```python
from build123d import *

# Parameters (mm, degrees)
SKETCH_1_R          = 1.6
EXTRUDE_1_DEPTH     = 3
SKETCH_5_W          = 8.427610272
SKETCH_5_H          = 29.562823711
CUT_EXTRUDE_4_DEPTH = 10
SKETCH_7_W          = 55.144779456
SKETCH_7_H          = 10
CUT_EXTRUDE_1_DEPTH = 100
CUT_EXTRUDE_5_DEPTH = 100
CUT_EXTRUDE_6_DEPTH = 100
FILLET_3_R          = 3
SKETCH_10_W         = 2
SKETCH_10_H         = 2
SKETCH_10_H_2       = 11
SKETCH_10_R         = 1.5
CUT_EXTRUDE_7_DEPTH = 10
SKETCH_11_R         = 11
CUT_EXTRUDE_8_DEPTH = 10


with BuildPart() as part:
    # 草图1 → 凸台-拉伸1 (new body)
    with BuildSketch(Plane(origin=(0, 0, 0), x_dir=(1, 0, 0), z_dir=(0, 1, 0))):
        Polygon((-1, -77.5), (-40, -77.5), (-40, -235.15), (110, -235.15), (110, -77.5), (71, -77.5), (71, -47.937176289), (113.89906921, -47.937176289), (113.89906921, 47.937176289), (71, 47.937176289), (71, 77.5), (110, 77.5), (110, 235.15), (-40, 235.15), (-40, 77.5), (-1, 77.5), (-1, 47.937176289), (-43.89906921, 47.937176289), (-43.89906921, -47.937176289), (-1, -47.937176289), align=None)
        with Locations(Location((48.025, -63.59, 0), (0, 0, 90))):
            Circle(SKETCH_1_R, mode=Mode.SUBTRACT)
        with Locations(Location((58.025, -63.59, 0), (0, 0, 90))):
            Circle(SKETCH_1_R, mode=Mode.SUBTRACT)
        with Locations(Location((58.025, 63.41, 0), (0, 0, 90))):
            Circle(SKETCH_1_R, mode=Mode.SUBTRACT)
        with Locations(Location((48.025, 63.41, 0), (0, 0, 90))):
            Circle(SKETCH_1_R, mode=Mode.SUBTRACT)
        with Locations(Location((11.975, -63.59, 0), (0, 0, 270))):
            Circle(SKETCH_1_R, mode=Mode.SUBTRACT)
        with Locations(Location((21.975, -63.59, 0), (0, 0, 270))):
            Circle(SKETCH_1_R, mode=Mode.SUBTRACT)
        with Locations(Location((21.975, 63.41, 0), (0, 0, 270))):
            Circle(SKETCH_1_R, mode=Mode.SUBTRACT)
        with Locations(Location((11.975, 63.41, 0), (0, 0, 270))):
            Circle(SKETCH_1_R, mode=Mode.SUBTRACT)
        with BuildLine():
            Line((30.075, -69.59), (30.075, -66.41))
            ThreePointArc((30.075, -66.41), (28.475, -64.81), (26.875, -66.41))
            Line((26.875, -66.41), (18.125, -66.41))
            ThreePointArc((18.125, -66.41), (16.525, -64.81), (14.925, -66.41))
            Line((14.925, -66.41), (14.925, -69.59))
            ThreePointArc((14.925, -69.59), (16.525, -71.19), (18.125, -69.59))
            Line((18.125, -69.59), (26.875, -69.59))
            ThreePointArc((26.875, -69.59), (28.475, -71.19), (30.075, -69.59))
        make_face(mode=Mode.SUBTRACT)
        with BuildLine():
            Line((43.125, 69.59), (51.875, 69.59))
            ThreePointArc((51.875, 69.59), (53.475, 71.19), (55.075, 69.59))
            Line((55.075, 69.59), (55.075, 66.41))
            ThreePointArc((55.075, 66.41), (53.475, 64.81), (51.875, 66.41))
            Line((51.875, 66.41), (43.125, 66.41))
            ThreePointArc((43.125, 66.41), (41.525, 64.81), (39.925, 66.41))
            Line((39.925, 66.41), (39.925, 69.59))
            ThreePointArc((39.925, 69.59), (41.525, 71.19), (43.125, 69.59))
        make_face(mode=Mode.SUBTRACT)
        with BuildLine():
            Line((55.075, -69.59), (55.075, -66.41))
            ThreePointArc((55.075, -66.41), (53.475, -64.81), (51.875, -66.41))
            Line((51.875, -66.41), (43.125, -66.41))
            ThreePointArc((43.125, -66.41), (41.525, -64.81), (39.925, -66.41))
            Line((39.925, -66.41), (39.925, -69.59))
            ThreePointArc((39.925, -69.59), (41.525, -71.19), (43.125, -69.59))
            Line((43.125, -69.59), (51.875, -69.59))
            ThreePointArc((51.875, -69.59), (53.475, -71.19), (55.075, -69.59))
        make_face(mode=Mode.SUBTRACT)
        with BuildLine():
            Line((14.925, 69.59), (14.925, 66.41))
            ThreePointArc((14.925, 66.41), (16.525, 64.81), (18.125, 66.41))
            Line((18.125, 66.41), (26.875, 66.41))
            ThreePointArc((26.875, 66.41), (28.475, 64.81), (30.075, 66.41))
            Line((30.075, 66.41), (30.075, 69.59))
            ThreePointArc((30.075, 69.59), (28.475, 71.19), (26.875, 69.59))
            Line((26.875, 69.59), (18.125, 69.59))
            ThreePointArc((18.125, 69.59), (16.525, 71.19), (14.925, 69.59))
        make_face(mode=Mode.SUBTRACT)
    extrude(amount=EXTRUDE_1_DEPTH)

    # 草图5 → 切除-拉伸4 (cut)
    with BuildSketch(Plane.XZ):
        with Locations((66.786194864, 62.718588145)):
            Rectangle(SKETCH_5_W, SKETCH_5_H)
        with Locations((3.213805136, 62.718588145)):
            Rectangle(SKETCH_5_W, SKETCH_5_H)
        with Locations((3.213805136, -62.718588145)):
            Rectangle(SKETCH_5_W, SKETCH_5_H)
        with Locations((66.786194864, -62.718588145)):
            Rectangle(SKETCH_5_W, SKETCH_5_H)
    extrude(amount=-CUT_EXTRUDE_4_DEPTH, mode=Mode.SUBTRACT)

    # 草图7 → 切除-拉伸-薄壁1 (cut)
    with BuildSketch(Plane(origin=(0, 0, 0), x_dir=(-1, 0, 0), z_dir=(0, -1, 0))):
        with Locations((-35, -55.277176289)):
            Rectangle(SKETCH_7_W, SKETCH_7_H)
        Polygon((-113.89906921, -0.33), (-113.89906921, 47.607176289), (-62.572389728, 47.607176289), (-62.572389728, 49.947176289), (-7.427610272, 49.947176289), (-7.427610272, 47.607176289), (43.89906921, 47.607176289), (43.89906921, -0.33), (33.89906921, -0.33), (33.89906921, 37.607176289), (-17.427610272, 37.607176289), (-17.427610272, 39.947176289), (-52.572389728, 39.947176289), (-52.572389728, 37.607176289), (-103.89906921, 37.607176289), (-103.89906921, -0.33), align=None)
    extrude(amount=-CUT_EXTRUDE_1_DEPTH, mode=Mode.SUBTRACT)


with BuildPart() as cut_extrude_1_piece_1:
    # of the separate pieces the step leaves, piece 1, a body of its own (cut_extrude_1_pieces)
    add(part.part.solids().sort_by_distance((7.427610272, 0, -77.5))[0])

    # 草图9 → 切除-拉伸6 (cut)
    with BuildSketch(Plane.XZ):
        Polygon((-40, -102.5), (110, -102.5), (124.211694431, -119.691261336), (154.987235789, -211.57345947), (124.211694431, -286.861832075), (-63.673505757, -270.701496299), (-75.556105593, -182.770257517), (-74.082044988, -165.632360403), align=None)
    extrude(amount=-CUT_EXTRUDE_6_DEPTH, mode=Mode.SUBTRACT)

    # 圆角3
    fillet_3_edges = [cut_extrude_1_piece_1.edges().sort_by_distance(p)[0] for p in [
        (110, 1.5, -77.5),
        (-40, 1.5, -77.5),
        (62.572389728, 1.5, -77.5),
        (7.427610272, 1.5, -77.5),
        (-40, 1.5, -102.5),
        (110, 1.5, -102.5),
        (7.427610272, 1.5, -49.947176289),
        (62.572389728, 1.5, -49.947176289),
    ]]
    fillet(fillet_3_edges, radius=FILLET_3_R)

    # 草图10 → 切除-拉伸7 (cut)
    with BuildSketch(Plane.XZ):
        with BuildLine():
            ThreePointArc((-35, -84.5), (-34, -83.5), (-35, -82.5))
            Line((-35, -82.5), (-35, -84.5))
        make_face()
        with BuildLine():
            Line((-37, -84.5), (-37, -82.5))
            ThreePointArc((-37, -82.5), (-38, -83.5), (-37, -84.5))
        make_face()
        with Locations((-36, -83.5)):
            Rectangle(SKETCH_10_W, SKETCH_10_H)
        with Locations((-36, -90)):
            Rectangle(SKETCH_10_W, SKETCH_10_H_2)
        with Locations((-36, -96.5)):
            Rectangle(SKETCH_10_W, SKETCH_10_H)
        with BuildLine():
            Line((-37, -97.5), (-37, -95.5))
            ThreePointArc((-37, -95.5), (-38, -96.5), (-37, -97.5))
        make_face()
        with BuildLine():
            ThreePointArc((-35, -97.5), (-34, -96.5), (-35, -95.5))
            Line((-35, -95.5), (-35, -97.5))
        make_face()
        with Locations(Location((-31.5, -95, 0), (0, 0, 270))):
            Circle(SKETCH_10_R)
        with Locations(Location((-31.5, -85, 0), (0, 0, 270))):
            Circle(SKETCH_10_R)
        with BuildLine():
            ThreePointArc((107, -97.5), (108, -96.5), (107, -95.5))
            Line((107, -95.5), (107, -97.5))
        make_face()
        with Locations((106, -96.5)):
            Rectangle(SKETCH_10_W, SKETCH_10_H)
        with BuildLine():
            Line((105, -97.5), (105, -95.5))
            ThreePointArc((105, -95.5), (104, -96.5), (105, -97.5))
        make_face()
        with Locations((106, -90)):
            Rectangle(SKETCH_10_W, SKETCH_10_H_2)
        with BuildLine():
            ThreePointArc((107, -84.5), (108, -83.5), (107, -82.5))
            Line((107, -82.5), (107, -84.5))
        make_face()
        with Locations((106, -83.5)):
            Rectangle(SKETCH_10_W, SKETCH_10_H)
        with BuildLine():
            Line((105, -84.5), (105, -82.5))
            ThreePointArc((105, -82.5), (104, -83.5), (105, -84.5))
        make_face()
        with Locations(Location((101.5, -85, 0), (0, 0, 270))):
            Circle(SKETCH_10_R)
        with Locations(Location((101.5, -95, 0), (0, 0, 270))):
            Circle(SKETCH_10_R)
    extrude(amount=-CUT_EXTRUDE_7_DEPTH, mode=Mode.SUBTRACT)

    # 草图11 → 切除-拉伸8 (cut)
    with BuildSketch(Plane.XZ):
        with Locations(Location((35, -86.015496457, 0), (0, 0, 270))):
            Circle(SKETCH_11_R)
    extrude(amount=-CUT_EXTRUDE_8_DEPTH, mode=Mode.SUBTRACT)


with BuildPart() as cut_extrude_1_piece_2:
    # of the separate pieces the step leaves, piece 2, a body of its own (cut_extrude_1_pieces)
    add(part.part.solids().sort_by_distance((-40, 0, 77.5))[0])


with BuildPart() as cut_extrude_1_piece_3:
    # of the separate pieces the step leaves, piece 3, a body of its own (cut_extrude_1_pieces)
    add(part.part.solids().sort_by_distance((7.427610272, 0, 50.277176289))[0])


with BuildPart() as cut_extrude_1_piece_4:
    # of the separate pieces the step leaves, piece 4, a body of its own (cut_extrude_1_pieces)
    add(part.part.solids().sort_by_distance((113.89906921, 0, -47.607176289))[0])


with BuildPart() as cut_extrude_1_piece_5:
    # of the separate pieces the step leaves, piece 5, a body of its own (cut_extrude_1_pieces)
    add(part.part.solids().sort_by_distance((-43.89906921, 0, -47.937176289))[0])


with BuildPart() as cut_extrude_5_tool:
    # 草图8 → 切除-拉伸5 (new body)
    with BuildSketch(Plane(origin=(0, 0, 0), x_dir=(-1, 0, 0), z_dir=(0, -1, 0))):
        Polygon((78.212914253, 60.385355647), (0, 54.326624312), (-4.481912928, 51.672567956), (-7.938908088, 48.761414138), (-49.331876445, 46.578048774), (-63.52375131, 48.761414138), (-79.080229528, 55.85735157), (-126.563695568, 60.385355647), (-136.561762242, 25.020008622), (-185.509289936, -177.467896247), (-114.798778659, -331.741539621), (230.896230576, -266.427705394), (230.896230576, -108.933419225), (223.681342993, -70.746247105), align=None)
    extrude(amount=-CUT_EXTRUDE_5_DEPTH)


with BuildPart() as cut_extrude_1_piece_2_1:
    add(cut_extrude_1_piece_2.part)

    # 切除-拉伸5: cut by cut_extrude_5_tool
    add(cut_extrude_5_tool.part, mode=Mode.SUBTRACT)


with BuildPart() as cut_extrude_1_piece_3_1:
    add(cut_extrude_1_piece_3.part)

    # 切除-拉伸5: cut by cut_extrude_5_tool
    add(cut_extrude_5_tool.part, mode=Mode.SUBTRACT)


with BuildPart() as cut_extrude_1_piece_4_1:
    add(cut_extrude_1_piece_4.part)

    # 切除-拉伸5: cut by cut_extrude_5_tool
    add(cut_extrude_5_tool.part, mode=Mode.SUBTRACT)


with BuildPart() as cut_extrude_1_piece_5_1:
    add(cut_extrude_1_piece_5.part)

    # 切除-拉伸5: cut by cut_extrude_5_tool
    add(cut_extrude_5_tool.part, mode=Mode.SUBTRACT)


solid = cut_extrude_1_piece_1.part
```
CAD build for the part. Positions are in the model's coordinates, mm. A direction names the side the tool comes from. Give positions to 0.01 mm unless a question says otherwise; leave off trailing zeros. Write each loop counter-clockwise with the first axis right and the second up, starting at its lowest first coordinate (ties: lowest second). Pieces come first, ordered by that corner, then holes. Notation, with made-up numbers: (-36, 25) -> (-23, 25) arc R27 cw to (-23, 56) -> close; hole circle Ø1 at (34.5, -7). An arc over 180 degrees is marked (long way). Write each question's results on one line, items separated by ' | '.
1. Drop flat-ended pins along their axis: P1, Ø1.6, axis at x = -36.5, y = 2, coming from the +Z side; P2, Ø1.5, axis at y = 1, z = -67.5, coming from the +X side; P3, Ø3, axis at x = 21.975, z = -63.41, coming from the +Y side; P4, Ø1.5, axis at y = 2, z = -68.5, coming from the -X side. Give the stop position or say it passes through.
Geometry check:
P1: z = -77.5 | P2: x = 62.57 | P3: through | P4: x = 7.43
2. Cut at B-B, the plane x = 101.5. Write the cut outline in (y, z), then the cut area to 3 significant figures.
Geometry check:
outline: (0, -102.5) -> (3, -102.5) -> (3, -96.5) -> (0, -96.5) -> close; (0, -93.5) -> (3, -93.5) -> (3, -86.5) -> (0, -86.5) -> close; (0, -83.5) -> (3, -83.5) -> (3, -77.5) -> (0, -77.5) -> close | area: 57.0 mm²
3. Which spindle directions (+Z, -Z, +X, -X, +Y, -Y) get a long thin tool onto all of the face, cutting with end or side? Do faces 1 (the flat face through (22, 1, -66.41)), 2 (the flat face through (7.428, 1, -64)), 3 (the cylindrical face through (109.1, 1.52, -101.64)). Say none if no direction does.
Geometry check:
face 1: +Y, -Y | face 2: +Z, -X, +Y, -Y | face 3: -Z, +X, +Y, -Y
4. Cut at A-A, the plane z = -63.41. Write the cut outline in (x, y) (3 decimals).
Geometry check:
outline: (7.428, 0) -> (10.375, 0) -> (10.375, 3) -> (7.428, 3) -> close; (13.575, 0) -> (20.375, 0) -> (20.375, 3) -> (13.575, 3) -> close; (23.575, 0) -> (46.425, 0) -> (46.425, 3) -> (23.575, 3) -> close; (49.625, 0) -> (56.425, 0) -> (56.425, 3) -> (49.625, 3) -> close; (59.625, 0) -> (62.572, 0) -> (62.572, 3) -> (59.625, 3) -> close
5. Cut at C-C, the plane z = -90. Write the cut outline in (x, y), then the cut area to 3 significant figures.
Geometry check:
outline: (-40, 0) -> (-37, 0) -> (-37, 3) -> (-40, 3) -> close; (-35, 0) -> (24.75, 0) -> (24.75, 3) -> (-35, 3) -> close; (45.25, 0) -> (105, 0) -> (105, 3) -> (45.25, 3) -> close; (107, 0) -> (110, 0) -> (110, 3) -> (107, 3) -> close | area: 376 mm²
6. Cut at D-D, the plane y = 2.35. Give the number of separate pieces and of enclosed holes in the cut face, then the cut area to 3 significant figures.
Geometry check:
separate pieces: 1 | enclosed holes: 13 | area: 4,620 mm²
7. Wall check: probe 1 along Z at (x, y) = (101.5, 1.45); probe 2 along X at (y, z) = (2.05, -63.41) (3 decimals); probe 3 along X at (y, z) = (1.9, -95). Give the ranges that are in metal, low to high. Write a range as [from, to].
Geometry check:
probe 1: [-102.5, -96.5], [-93.5, -86.5], [-83.5, -77.5] | probe 2: [7.428, 10.375], [13.575, 20.375], [23.575, 46.425], [49.625, 56.425], [59.625, 62.572] | probe 3: [-40, -37], [-35, -33], [-30, 28.65], [41.35, 100], [103, 105], [107, 110]
8. Two-plate mould, pull along Z, no slides. Class faces 4 (the cylindrical face through (-39.14, 1.52, -78.4)), 5 (the flat face through (-35, 1, -90)), 6 (the flat face through (107, 1, -90)), 7 (the flat face through (110, 1, -90)): pulls with the +Z half, pulls with the -Z half, needs draft (parallel to the pull), parting line crosses it, or undercut.
Geometry check:
face 4: pulls with the +Z half | face 5: undercut | face 6: undercut | face 7: needs draft
